from build123d import *

# Parameters (mm, degrees)
F0_W     = 384.175
F0_H     = 609.6
F1_DEPTH = 914.4
F2_T     = -12.7
F3_W     = 384.175
F3_H     = 914.4
F3_W_2   = 368.3
F3_H_2   = 901.7
F3_W_3   = 358.775
F3_H_3   = 889
F3_W_4   = 301.625
F3_H_4   = 831.85
F4_DEPTH = 19.05
F3_W_5   = 254
F3_H_5   = 787.4
F5_DEPTH = 19.05
F6_W     = 254
F6_H     = 7.9375
F7_DEPTH = 787.4
F8_SIZE  = 3.175


with BuildPart() as f1:
    # F0 (on Top) → F1 (new body)
    with BuildSketch(Plane.XY):
        Rectangle(F0_W, F0_H)
    extrude(amount=F1_DEPTH)

    # F2
    f2_openings = [f1.faces().sort_by_distance(p)[0] for p in [
        (0, -304.8, 457.2),
    ]]
    offset(amount=F2_T, openings=f2_openings)

    # F3 (on face) → F4 (join)
    with BuildSketch(Plane.XZ.offset(304.8)):
        with Locations((0, 457.2)):
            Rectangle(F3_W, F3_H)
        with Locations((0, 457.2)):
            Rectangle(F3_W_2, F3_H_2, mode=Mode.SUBTRACT)
        with Locations((0, 457.2)):
            Rectangle(F3_W_3, F3_H_3)
        with Locations((0, 457.2)):
            Rectangle(F3_W_4, F3_H_4, mode=Mode.SUBTRACT)
    extrude(amount=-F4_DEPTH)

    # F3 (on face) → F5 (join)
    with BuildSketch(Plane.XZ.offset(304.8)):
        with Locations((0, 457.2)):
            Rectangle(F3_W_3, F3_H_3)
        with Locations((0, 457.2)):
            Rectangle(F3_W_4, F3_H_4, mode=Mode.SUBTRACT)
        with Locations((0, 457.2)):
            Rectangle(F3_W_4, F3_H_4)
        with Locations((0, 457.2)):
            Rectangle(F3_W_5, F3_H_5, mode=Mode.SUBTRACT)
    extrude(amount=F5_DEPTH)

    # F6 (on face) → F7 (join, through all)
    with BuildSketch(Plane(origin=(0, 0, 850.9), x_dir=(1, 0, 0), z_dir=(0, 0, -1))):
        with Locations((0, 313.53125)):
            Rectangle(F6_W, F6_H)
    extrude(amount=F7_DEPTH)

    # F8
    f8_edges = [f1.edges().sort_by_distance(p)[0] for p in [
        (0, -323.85, 63.5),
        (-127, -323.85, 457.2),
        (127, -323.85, 457.2),
        (0, -323.85, 850.9),
        (-192.0875, 304.8, 457.2),
    ]]
    chamfer(f8_edges, length=F8_SIZE)


solid = f1.part
Check sheet for the modelled part. Datum: model origin and axes. Units: mm. A direction names the side the tool comes from. Round coordinates to 2 decimals unless told otherwise and drop trailing zeros. Loops run counter-clockwise (first coordinate to the right, second up) from the corner with the lowest first, then second, coordinate; pieces in that order, holes last. Notation, with made-up numbers: M 72,69.5 L 80,69.5 A10 ccw 80,73.5 Z; hole C -0.5,0 d9. An arc over 180 degrees is marked long. One line per item, written item: value.
(1) Sectioned sample at A-A, the plane y = -33.5. Record the cut outline in (x, z), then the cut area to 3 significant figures.
Computed values:
outline: M -192.09,0 L 192.09,0 L 192.09,914.4 L -192.09,914.4 Z; hole M -179.39,12.7 L 179.39,12.7 L 179.39,901.7 L -179.39,901.7 Z
area: 32,300 mm^2
(2) Thickness scan on line 1 (X direction, y = 179, z = 137); line 2 (Z direction, x = 55.5, y = -135); line 3 (Y direction, x = 163, z = 372). Record the ranges inside material, lowest first.
Computed values:
line 1: x = -192.09 to -179.39, 179.39 to 192.09
line 2: z = 0 to 12.7, 901.7 to 914.4
line 3: y = -323.85 to -285.75, 292.1 to 304.8
(3) Release check for a two-part mould opening along Y. For faces 4 (the face through (-2, -317.5, 463)), 5 (the face through (-3, 292.1, 451)), 6 (the face through (-2, -295, 41.275)), 7 (the face through (-3, -314, 12.7)) record: +Y half, -Y half, draft (parallel to the pull), parting line (faces both ways), or undercut.
Computed values:
face 4: -Y half
face 5: undercut
face 6: undercut
face 7: draft
(4) Access from +Z, -Z, +X, -X, +Y, -Y to the whole of each face (thin tool, end or side, straight path). Record for faces 1 (the face through (-179.388, -1, 451)), 2 (the face through (-179.388, -314, 451)), 3 (the face through (-3, -314, 901.7)).
Computed values:
face 1: none
face 2: +Z, -Z, -X, -Y
face 3: +Z, +X, -X, -Y
(5) Depth check by flat-ended pin: pin 1 Ø4 at (x, z) = (-88, 156) entering from -Y; pin 2 Ø1 at (x, y) = (13.5, -319.5) entering from +Z; pin 3 Ø2.5 at (x, y) = (60.5, -319) entering from -Z. Enter the tip coordinate at first touch or a pass-through.
Computed values:
pin 1: stops at y = -317.5
pin 2: stops at z = 901.7
pin 3: stops at z = 12.7
